Here's the drawing with two shaded views (mm, measured from the low corner). I have some questions. A direction names the side the tool comes from. Coordinates: 2 decimals unless noted, no trailing zeros. Order: outer loops, then holes, each group sorted by start corner. A loop starts at its lowest first (then second) coordinate and runs counter-clockwise, first axis right, second up. Notation, with made-up numbers: (33, 49) -> (56, 49) arc R10 ccw to (56, 68) -> close; hole circle Ø10 at (-6.5, 6.5). An arc over 180 degrees is marked (long way). Answer as a JSON object with one key per item and string values. Group by question number.
(1) If we mould it in two halves opening along Y, with no side actions, what happens to the marked faces 1, 2 and 3? For each: pulls with the +Y half, pulls with the -Y half, needs draft (parallel to the pull), parting line crosses it, or undercut.
(2) I want a section at A-A, the plane x = 19.25. List the corners of the cut face in (y, z) for me (1 decimal).
(3) I want a section at C-C, the plane x = 8.75. List the corners of the cut face in (y, z) for me.
(4) I need wall thicknesses on line 1 (X direction, y = 14.5, z = 14.25); line 2 (X direction, y = 2, z = 8.75); line 3 (Z direction, x = 21, y = 4.75) (1 decimal). Which ranges of each line are inside material? Lowest first, please.
(5) I want a section at D-D, the plane x = 15. List the corners of the cut face in (y, z) for me.
(6) For pin 1 (2 mm diameter, centred on x = 17.5, z = 7, fed in from +Y); pin 2 (3 mm diameter, centred on y = 5.5, z = 4.5, fed in from +X); pin 3 (10 mm diameter, centred on x = 13.5, z = 16.5, fed in from -Y), each with a flat end and sliding along its axis, tell me the tip position at first contact or that it passes through.
(7) Which directions (+Z, -Z, +X, -X, +Y, -Y) give clear straight access to the entire face, cutting with the end or side of a thin tool? Please do the marked faces 4, 5 and 6.
(8) I want a section at B-B, the plane x = 26.25. List the corners of the cut face in (y, z) for me (1 decimal).
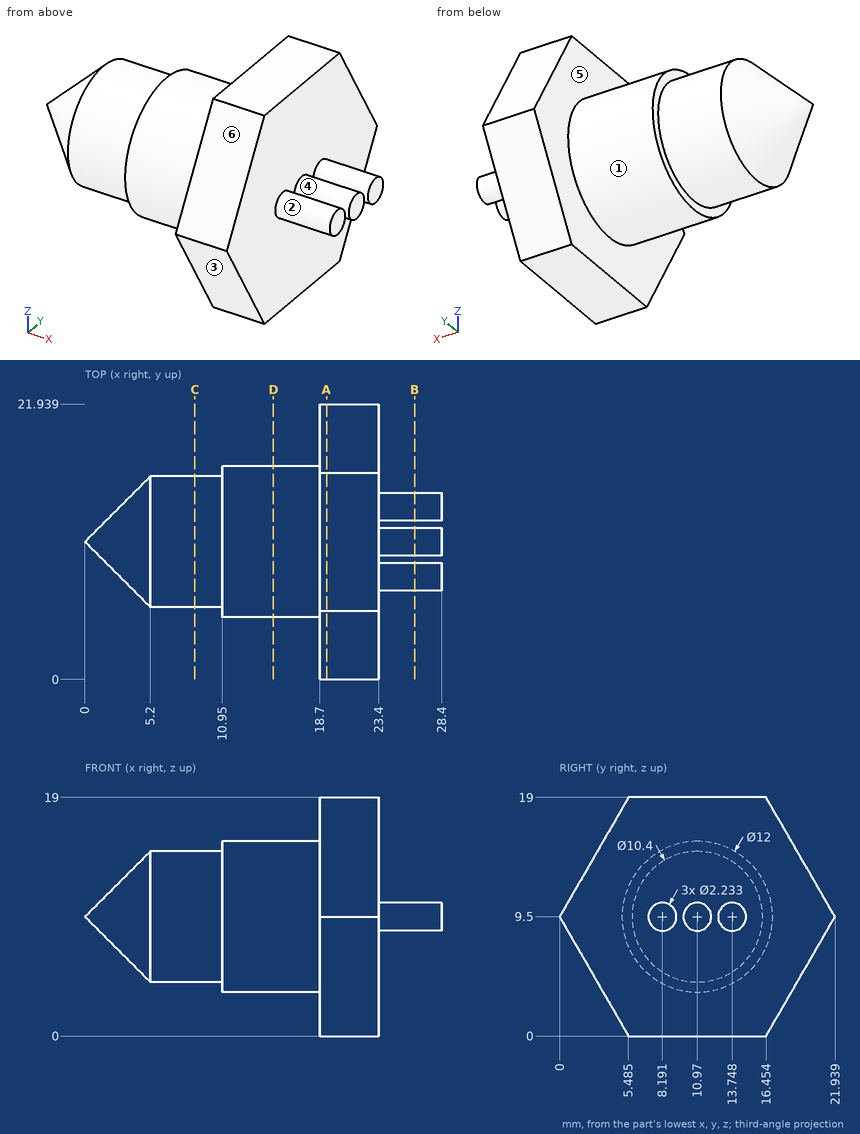
Computed values:
{
 "1": {"face 1": "parting line crosses it", "face 2": "undercut", "face 3": "pulls with the -Y half"},
 "2": {"outline": "(0, 9.5) -> (5.5, 0) -> (16.5, 0) -> (21.9, 9.5) -> (16.5, 19) -> (5.5, 19) -> close"},
 "3": {"outline": "circle Ø10.4 at (10.97, 9.5)"},
 "4": {"line 1": "x = 10.95 to 23.4", "line 2": "x = 18.7 to 23.4", "line 3": "z = 1.3 to 17.7"},
 "5": {"outline": "circle Ø12 at (10.97, 9.5)"},
 "6": {"pin 1": "stops at y = 16.78", "pin 2": "stops at x = 23.4", "pin 3": "stops at y = 5.31"},
 "7": {"face 4": "+X", "face 5": "-X", "face 6": "+Z, +X, -X, -Y"},
 "8": {"outline": "circle Ø2.2 at (8.2, 9.5); circle Ø2.2 at (11, 9.5); circle Ø2.2 at (13.7, 9.5)"}
}
